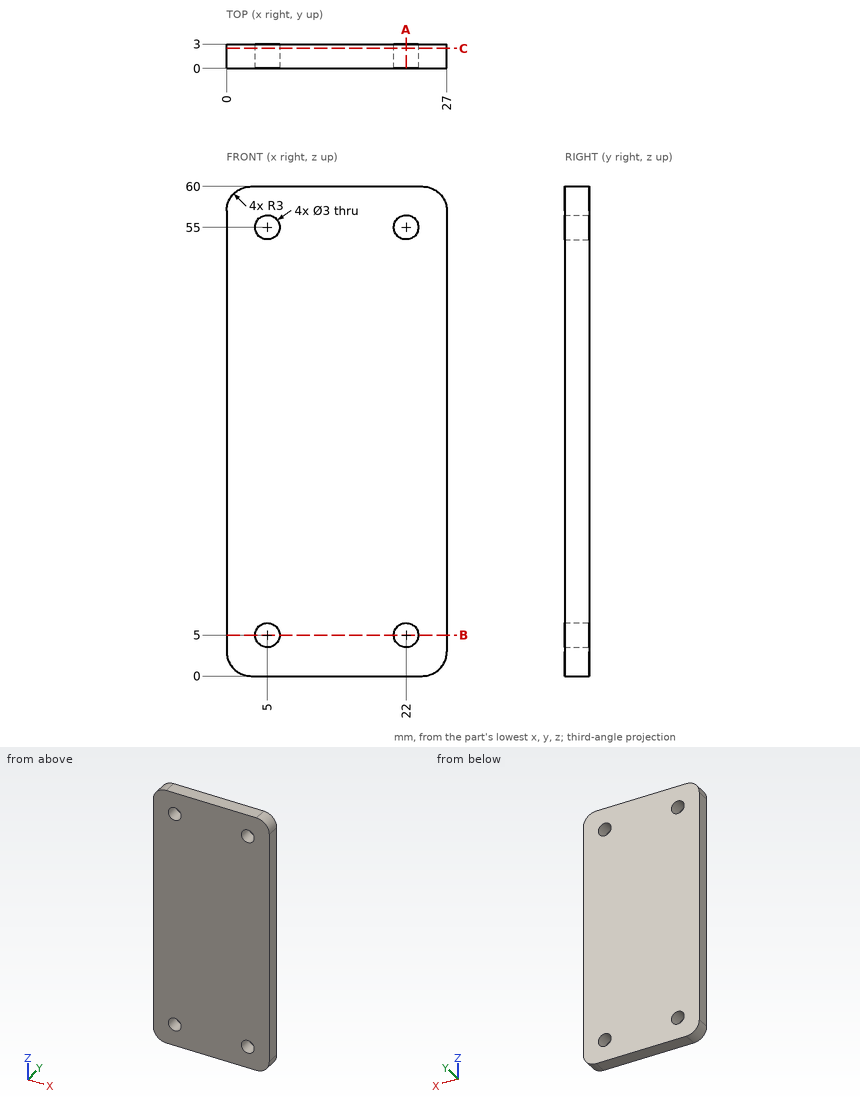
Job drawing, mm, ordinate dimensions from the low corner. One solid piece. Round coordinates to 2 decimals unless told otherwise and drop trailing zeros. Write each loop counter-clockwise with the first axis right and the second up, starting at its lowest first coordinate (ties: lowest second). Pieces come first, ordered by that corner, then holes. Notation, with made-up numbers: M 28,59.5 L 65,59.5 A17 cw 65,83.5 Z; hole C 8,16.5 d3. An arc over 180 degrees is marked long. Return JSON: item names as keys, results as strings. Group by question number.
(1) Saw through at B-B on z = 5. Write the cut outline in (x, y), then the cut area to 3 significant figures.
(2) Saw through at C-C on y = 2.45. Write the cut outline in (x, z), then the cut area to 3 significant figures.
(3) Drill centre lines: probe 1 along X at (y, z) = (2.3, 5); probe 2 along Z at (x, y) = (5, 1.45); probe 3 along Z at (x, y) = (5.5, 2). Where is each one in solid material? Low to high.
(4) Pin check, flat tip, straight feed: pin 1 Ø2.5 at (x, z) = (22, 5) entering from -Y. Stop position of the tip, or through.
(5) Saw through at A-A on x = 22. Write the cut outline in (y, z), then the cut area to 3 significant figures.
Returned:
{
 "1": {"outline": "M 0,0 L 3.5,0 L 3.5,3 L 0,3 Z; M 6.5,0 L 20.5,0 L 20.5,3 L 6.5,3 Z; M 23.5,0 L 27,0 L 27,3 L 23.5,3 Z", "area": "63.0 mm²"},
 "2": {"outline": "M 0,3 A3 ccw 3,0 L 24,0 A3 ccw 27,3 L 27,57 A3 ccw 24,60 L 3,60 A3 ccw 0,57 Z; hole C 5,5 d3; hole C 5,55 d3; hole C 22,5 d3; hole C 22,55 d3", "area": "1,580 mm²"},
 "3": {"probe 1": "0 to 3.5, 6.5 to 20.5, 23.5 to 27", "probe 2": "0 to 3.5, 6.5 to 53.5, 56.5 to 60", "probe 3": "0 to 3.59, 6.41 to 53.59, 56.41 to 60"},
 "4": {"pin 1": "through"},
 "5": {"outline": "M 0,0 L 3,0 L 3,3.5 L 0,3.5 Z; M 0,6.5 L 3,6.5 L 3,53.5 L 0,53.5 Z; M 0,56.5 L 3,56.5 L 3,60 L 0,60 Z", "area": "162 mm²"}
}
